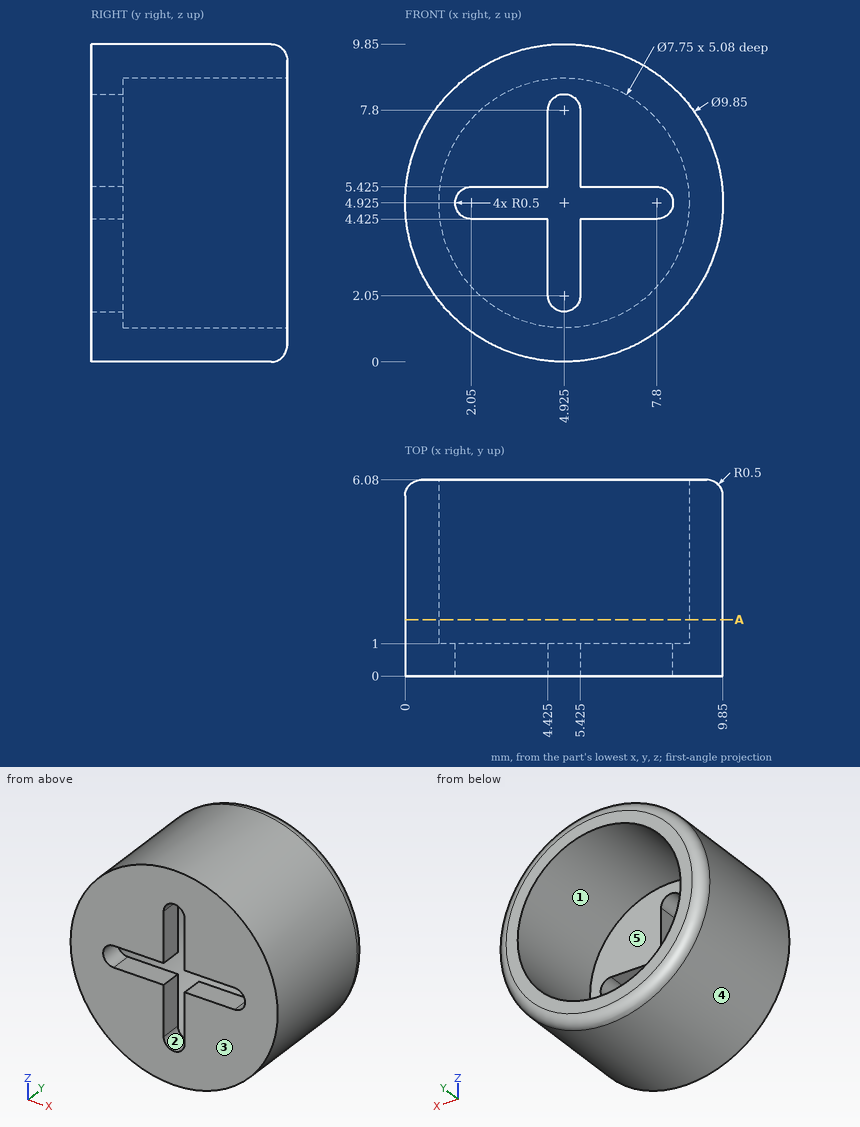
Source: three-view drawing plus pictorial views. Frame: mm from the lowest corner of the part. A direction names the side the tool comes from. Give positions to 0.01 mm unless a question says otherwise; leave off trailing zeros. Write each loop counter-clockwise with the first axis right and the second up, starting at its lowest first coordinate (ties: lowest second). Pieces come first, ordered by that corner, then holes. Notation, with made-up numbers: M -24.75,24 L 34.25,24 A27 cw 34.25,52 Z; hole C 80.25,72 d6. An arc over 180 degrees is marked long. Use one line per item in the form item = value.
1. Ray query, L1, parallel to X at y = 5, z = 5; L2, parallel to Y at x = 5.75, z = 2.75; L3, parallel to X at y = 3.25, z = 3. Return the intervals inside material, ascending.
Outcome:
L1 = 0 to 1.05, 8.8 to 9.85
L2 = 0 to 1
L3 = 0.39 to 1.56, 8.29 to 9.46
2. Reachability of the marked faces 1 and 2 from +Z, -Z, +X, -X, +Y, -Y: full face, straight path, thin tool, end or side. Return the list, or none.
Outcome:
face_1 = +Y
face_2 = +Y, -Y
3. Cut plane A-A on y = 1.75. Return loops of the section in (x, z) (3 decimals).
Outcome:
outline = C 4.925,4.925 d9.85; hole C 4.925,4.925 d7.75
4. First-contact query: P1, Ø1.1, axis at y = 0.5, z = 7, coming from the -X side; P2, Ø0.8, axis at x = 3.5, y = 0.5, coming from the +Z side; P3, Ø1.1, axis at y = 0.5, z = 6, coming from the +X side. Flat tips, straight axial feed; report the tip coordinate or a pass-through.
Outcome:
P1 = 0.24
P2 = 9.74
P3 = 9.82
5. Mould query, pull axis Z, two halves, no side actions, for the marked faces 3, 4 and 5. Classes: released by +Z, released by -Z, zero draft, split by the parting line, or undercut.
Outcome:
face_3 = zero draft
face_4 = split by the parting line
face_5 = undercut
